Design review of the part built by this model. Coordinates are the model's own, in mm. A direction names the side the tool comes from. Round coordinates to 2 decimals unless told otherwise and drop trailing zeros. Loops run counter-clockwise (first coordinate to the right, second up) from the corner with the lowest first, then second, coordinate; pieces in that order, holes last. Notation, with made-up numbers: (69.25, 58) - (127.25, 58) arc R20 ccw to (127.25, 75) - close; hole circle Ø4 at (76, 59.25). An arc over 180 degrees is marked (long way). Return JSON: item names as keys, results as strings. Group by question number.
from build123d import *

# Parameters (mm, degrees)
SKETCH1_W = 6.85
SKETCH1_H = 3.9


with BuildPart() as part:
    # Sketch1 → Revolve1 (revolve)
    with BuildSketch(Plane.XY, mode=Mode.PRIVATE) as revolve1_sk:
        Polygon((20.65, 5), (-20.65, 5), (-20.65, 3.9), (-20.65, 0), (20.65, 0), (20.65, 3.9), align=None)
        with Locations((-24.075, 1.95)):
            Rectangle(SKETCH1_W, SKETCH1_H)
        with Locations((24.075, 1.95)):
            Rectangle(SKETCH1_W, SKETCH1_H)
    revolve(revolve1_sk.sketch.rotate(Axis((-27.5, 0, 0), (1, 0, 0)), 90), axis=Axis((-27.5, 0, 0), (1, 0, 0)))


solid = part.part
Q1. Insertion check: pin 1 Ø1.5 at (x, z) = (0, 2.5) entering from +Y; pin 2 Ø1.5 at (x, z) = (-11, 1.5) entering from -Y; pin 3 Ø3 at (x, y) = (-5.5, -3.5) entering from -Z. Each pin has a flat end and moves straight along its axis. Give the tip position at first contact, or say it passes through.
Q2. Tool access review of faces 1 (the cylindrical face through (-24.03, -2.64, -2.87)), 2 (the cylindrical face through (24.12, -2.64, -2.87)), 3 (the flat face through (27.5, 0, 0)): name each direction out of +Z, -Z, +X, -X, +Y, -Y from which nothing blocks a thin tool from reaching the whole face with its end or side.
Q3. For line 1 (X direction, y = 3, z = -3.75); line 2 (Y direction, x = 15, z = 0.25); line 3 (Y direction, x = 11.5, z = 3.5), list the stretches that pass through material, from the lowest coordinate up.
Q4. Add section A-A, the plane y = 0. State the section outline as (x, z) points, plus the area to 3 significant figures.
Q5. Add section C-C, the plane x = 17. State the section outline as (y, z) points, plus the area to 3 significant figures.
Evaluation:
{
 "1": {"pin 1": "y = 4.68", "pin 2": "y = -4.94", "pin 3": "z = -4.58"},
 "2": {"face 1": "-X", "face 2": "+X", "face 3": "+Z, -Z, +X, +Y, -Y"},
 "3": {"line 1": "-20.65 to 20.65", "line 2": "-4.99 to 4.99", "line 3": "-3.57 to 3.57"},
 "4": {"outline": "(-27.5, -3.9) - (-20.65, -3.9) - (-20.65, -5) - (20.65, -5) - (20.65, -3.9) - (27.5, -3.9) - (27.5, 3.9) - (20.65, 3.9) - (20.65, 5) - (-20.65, 5) - (-20.65, 3.9) - (-27.5, 3.9) - close", "area": "520 mm²"},
 "5": {"outline": "circle Ø10 at (0, 0)", "area": "78.5 mm²"}
}
